Model file for the job. Use its own axes, mm. A direction names the side the tool comes from. Round coordinates to 2 decimals unless told otherwise and drop trailing zeros. Order: outer loops, then holes, each group sorted by start corner. A loop starts at its lowest first (then second) coordinate and runs counter-clockwise, first axis right, second up. Notation, with made-up numbers: (67, 57) -> (124, 57) arc R11 ccw to (124, 68) -> close; hole circle Ø10 at (-25.5, -33.5). An arc over 180 degrees is marked (long way). Put each result on its own line as item: value. Start each with the question number.
Q1. Cut at B-B, the plane z = 65.5. List the corners of the cut face in (x, y), and give its area (3 significant figures).
Q2. Probe L1, parallel to X at y = 1.9, z = 102; L2, parallel to X at y = 3.9, z = 28; L3, parallel to X at y = 3.2, z = 30. List the from-to ranges inside material, lowest first.
Q3. 3-axis set-ups, long thin cutter, end or side, ignore diameter. For faces 1 (the face through (-68, 2, 103.42)), 2 (the face through (-9.322, 2, 33)), 3 (the face through (-12.03, 2.46, 62.26)): which of +Z, -Z, +X, -X, +Y, -Y reach the whole face in a straight line?
Q4. Flat gauge pins, fed straight in: P1, Ø1, axis at x = -29.5, y = 4.5, coming from the +Z side; P2, Ø1.8, axis at y = 2, z = 109.5, coming from the +X side; P3, Ø1, axis at y = 2.5, z = 110, coming from the -X side. Where does each tip first touch, or does it go through?
Q5. Pull direction X, two halves, no side cores. Call faces 4 (the face through (-67.7, 2.46, 113.81)), 5 (the face through (-57.123, 2.465, 114.506)), 6 (the face through (-74.334, 2.465, 116.045)): released by +X, released by -X, zero draft, split by the parting line, or undercut.
Q6. Cut at A-A, the plane x = -20. List the corners of the cut face in (y, z), and give its area (3 significant figures).
Q7. Cut at C-C, the plane y = 1.9. State how many separate pieces and enclosed holes the cut face has, and give its area (3 significant figures).
from build123d import *

# Parameters (mm, degrees)
SKETCH2_R           = 3.0000000000000018
SKETCH2_R_2         = 1.4999999999993736
SKETCH2_R_3         = 1.5000000000000009
SKETCH2_R_4         = 1.4999999999993723
BOSS_EXTRUDE1_DEPTH = 5
FILLET1_R           = 1.5
FILLET3_R           = 10
FILLET5_R           = 10
CHAMFER1_SIZE       = 4.5
FILLET6_R           = 6
FILLET7_R           = 4
FILLET8_R           = 2
FILLET9_R           = 30
FILLET10_R          = 1


with BuildPart() as part:
    # Sketch2 → Boss-Extrude1 (new body)
    with BuildSketch(Plane(origin=(0, 0, 0), x_dir=(1, 0, 0), z_dir=(0, 1, 0))):
        with BuildLine():
            Line((-46.189355852298796, -96.42025186017804), (-39.496927389393186, -89.72782339727232))
            Line((-39.496927389393186, -89.72782339727232), (17.913506363615255, -32.31738964426288))
            Line((17.913506363615255, -32.31738964426288), (24.678224989376695, -32.31738964426288))
            Line((24.678224989376695, -32.31738964426288), (24.678224989376428, -17.06738964426295))
            Line((24.678224989376428, -17.06738964426295), (-7.595965049770856, -17.06738964426337))
            Line((-7.595965049770856, -17.06738964426337), (-7.595965049770857, -24.067389644263372))
            Line((-7.595965049770857, -24.067389644263372), (-9.321775010623746, -27.06012368042446))
            Line((-9.321775010623746, -27.06012368042446), (-9.32177501062375, -37.06738964426337))
            Line((-9.32177501062375, -37.06738964426337), (-9.321775010623757, -42.58210827002507))
            Line((-9.321775010623753, -42.58210827002507), (-54.6598701272448, -87.9202033866469))
            Line((-54.6598701272448, -87.9202033866469), (-60.17458875300816, -87.92020338664692))
            ThreePointArc((-60.17458875300816, -87.92020338664692), (-63.00301587775435, -89.09177626190073), (-64.17458875300817, -91.92020338664692))
            Line((-64.17458875300817, -91.92020338664692), (-64.17458875300817, -97.92020338664689))
            Line((-64.17458875300817, -97.92020338664689), (-70.17458875301077, -97.92020338664689))
            ThreePointArc((-70.17458875301077, -97.92020338664689), (-72.6339398041774, -98.76558892412923), (-74.05374095021992, -100.9444071830841))
            Line((-74.05374095021992, -100.9444071830841), (-77.14515150148509, -113.23391188563446))
            Line((-77.14515150148509, -113.23391188563446), (-71.4882972519927, -118.89076613512684))
            Line((-71.4882972519927, -118.89076613512684), (-59.047429208957894, -115.75810794021132))
            ThreePointArc((-59.047429208957894, -115.75810794021132), (-56.9723521770992, -114.3172183869977), (-56.174588753010745, -111.92020338664949))
            Line((-56.174588753010745, -111.92020338664949), (-56.174588753010745, -105.92020338664949))
            Line((-56.174588753010745, -105.92020338664949), (-50.174588753008145, -105.92020338664949))
            ThreePointArc((-50.174588753008145, -105.92020338664949), (-47.34616162826196, -104.74863051139567), (-46.174588753008145, -101.92020338664949))
            Line((-46.174588753008145, -101.92020338664949), (-46.17464642427909, -101.89872393503671))
            Line((-46.17464642427909, -101.89872393503671), (-46.189355852298796, -96.42025186017804))
        make_face()
        Polygon((-70.26446914062754, -114.4577399969996), (-72.71257361922765, -112.00963551839949), (-71.33075600396296, -106.51639746436214), (-66.89210317428027, -106.51639746436214), (-64.77078283072062, -108.63771780792177), (-64.7707828307206, -113.0744087552009), align=None, mode=Mode.SUBTRACT)
        with BuildLine():
            ThreePointArc((-61.67458875301074, -108.42020338664949), (-60.17458875301075, -106.92020338664949), (-58.67458875301077, -108.42020338664949))
            Line((-58.67458875301077, -108.42020338664949), (-58.674588753010774, -111.92020338664949))
            ThreePointArc((-58.674588753010774, -111.92020338664949), (-60.17458875301075, -113.42020338664946), (-61.67458875301073, -111.92020338664949))
            Line((-61.67458875301073, -111.92020338664949), (-61.67458875301074, -108.42020338664949))
        make_face(mode=Mode.SUBTRACT)
        with BuildLine():
            ThreePointArc((-66.67458875301074, -100.42020338664692), (-65.17458875301071, -101.92020338664692), (-66.67458875301074, -103.42020338664692))
            Line((-66.67458875301074, -103.42020338664692), (-70.17458875301077, -103.42020338664692))
            ThreePointArc((-70.17458875301077, -103.42020338664692), (-71.67458875301075, -101.92020338664692), (-70.17458875301077, -100.42020338664692))
            Line((-70.17458875301077, -100.4202033866469), (-66.67458875301074, -100.4202033866469))
        make_face(mode=Mode.SUBTRACT)
        with Locations(Location((-60.174588753008145, -101.92020338664949, 0), (0, 0, 270))):
            Circle(SKETCH2_R, mode=Mode.SUBTRACT)
        with BuildLine():
            ThreePointArc((-53.67458875300815, -103.42020338664949), (-55.17458875300815, -101.92020338664949), (-53.67458875300815, -100.42020338664949))
            Line((-53.67458875300815, -100.42020338664949), (-50.174588753008145, -100.42020338664949))
            ThreePointArc((-50.174588753008145, -100.42020338664949), (-48.67458875300816, -101.92020338664949), (-50.174588753008145, -103.42020338664949))
            Line((-50.174588753008145, -103.42020338664949), (-53.67458875300815, -103.42020338664949))
        make_face(mode=Mode.SUBTRACT)
        with BuildLine():
            ThreePointArc((-58.67458875300815, -95.42020338664692), (-60.17458875300815, -96.9202033866469), (-61.67458875300815, -95.42020338664692))
            Line((-61.674588753008145, -95.42020338664692), (-61.67458875300816, -91.92020338664692))
            ThreePointArc((-61.67458875300816, -91.92020338664692), (-60.174588753008145, -90.42020338664689), (-58.67458875300813, -91.92020338664692))
            Line((-58.67458875300813, -91.92020338664692), (-58.674588753008145, -95.42020338664692))
        make_face(mode=Mode.SUBTRACT)
        with Locations(Location((-1.1783767284213562, -42.92399136206118, 0), (0, 0, 270))):
            Circle(SKETCH2_R_2, mode=Mode.SUBTRACT)
        with Locations(Location((-3.3217750106237407, -28.067389644263372, 0), (0, 0, 270))):
            Circle(SKETCH2_R_3, mode=Mode.SUBTRACT)
        with Locations(Location((9.428224989376764, -32.31738964426288, 0), (0, 0, 270))):
            Circle(SKETCH2_R_4, mode=Mode.SUBTRACT)
        Polygon((1.0820753752795897, -25.575281589539195), (-1.459873180493811, -22.79599601598655), (-1.4598731804937872, -21.06738964426295), (17.849797864630506, -21.06738964426295), (11.740910030340089, -27.17627747855337), (10.272484798754686, -26.22755837455273), align=None, mode=Mode.SUBTRACT)
    extrude(amount=BOSS_EXTRUDE1_DEPTH)

    # Fillet1
    # the kernel refuses this fillet: 1.5 mm, written as the material it adds along each edge
    with BuildSketch(Plane(origin=(1.0820753752795897, 0, 25.575281589539195), x_dir=(0.9974908468725838, 0, 0.07079555357093803), z_dir=(0, 1, 0))) as fillet1_piece_1:
        with BuildLine():
            CenterArc((FILLET1_R * 0.398900109333, FILLET1_R), FILLET1_R, 226.50587582859146, 43.4941241714086)
            Line((-FILLET1_R * 0.289380073746, FILLET1_R * 0.274555040282), (0, 0))
            Line((0, 0), (FILLET1_R * 0.398900109333, 0))
        make_face()
    extrude(amount=5)
    with BuildSketch(Plane(origin=(-1.459873180493811, 0, 22.79599601598655), x_dir=(1.372e-14, 0, -1), z_dir=(0, 1, 0))) as fillet1_piece_2:
        with BuildLine():
            CenterArc((FILLET1_R * 0.388338270451, -FILLET1_R), FILLET1_R, 89.99999999999997, 42.44619337739144)
            Line((-FILLET1_R * 0.286559260205, -FILLET1_R * 0.262088539786), (0, 0))
            Line((0, 0), (FILLET1_R * 0.388338270451, 0))
        make_face()
    extrude(amount=5)
    with BuildSketch(Plane(origin=(-1.459873180493787, 0, 21.06738964426295), x_dir=(1, 0, 0), z_dir=(0, 1, 0))) as fillet1_piece_3:
        with BuildLine():
            CenterArc((FILLET1_R, -FILLET1_R), FILLET1_R, 90, 89.99999999999918)
            Line((-2.087e-14, -FILLET1_R), (0, 0))
            Line((0, 0), (FILLET1_R, 0))
        make_face()
    extrude(amount=5)
    with BuildSketch(Plane(origin=(11.740910030340089, 0, 27.17627747855337), x_dir=(-0.839945220222329, 0, -0.5426711960530642), z_dir=(0, 1, 0))) as fillet1_piece_4:
        with BuildLine():
            CenterArc((FILLET1_R * 0.807844840446, -FILLET1_R), FILLET1_R, 89.99999999999994, 77.86566453571226)
            Line((-FILLET1_R * 0.169812603282, -FILLET1_R * 0.789795521639), (0, 0))
            Line((0, 0), (FILLET1_R * 0.807844840446, -3e-17))
        make_face()
    extrude(amount=5)
    with BuildSketch(Plane(origin=(17.849797864630506, 0, 21.06738964426295), x_dir=(-0.7071067811865475, 0, 0.7071067811865475), z_dir=(0, 1, 0))) as fillet1_piece_5:
        with BuildLine():
            CenterArc((FILLET1_R * 2.41421356237, -FILLET1_R), FILLET1_R, 89.99999999999994, 135.00000000000006)
            Line((FILLET1_R * 1.70710678119, -FILLET1_R * 1.70710678119), (0, 0))
            Line((0, 0), (FILLET1_R * 2.41421356237, 1e-17))
        make_face()
    extrude(amount=5)
    # the kernel refuses this fillet: 1.5 mm, written as the material it takes off along each edge
    with BuildSketch(Plane(origin=(10.27248479875469, -0.9630450228974294, 26.22755837455273), x_dir=(0.8399452202223279, 0, 0.5426711960530661), z_dir=(0, 1, 0))) as fillet1_2_piece_1:
        with BuildLine():
            CenterArc((FILLET1_R * 0.256812006106, -FILLET1_R), FILLET1_R, 90.00000000000006, 28.805982084511456)
            Line((-FILLET1_R * 0.225033157983, -FILLET1_R * 0.123743623222), (0, 0))
            Line((0, 0), (FILLET1_R * 0.256812006106, 2e-17))
        make_face()
    extrude(amount=6.92609004579486, mode=Mode.SUBTRACT)

    # Fillet3
    fillet3_edges = [part.edges().sort_by_distance(p)[0] for p in [
        (17.913506363615255, 2.5, 32.31738964426288),
    ]]
    fillet(fillet3_edges, radius=FILLET3_R)

    # Fillet5
    fillet5_edges = [part.edges().sort_by_distance(p)[0] for p in [
        (-9.321775010623755, 2.5, 42.58210827002507),
    ]]
    fillet(fillet5_edges, radius=FILLET5_R)

    # Chamfer1
    chamfer1_edges = [part.edges().sort_by_distance(p)[0] for p in [
        (-64.17458875300817, 2.5, 97.92020338664689),
        (-56.174588753010745, 2.5, 105.92020338664949),
    ]]
    chamfer(chamfer1_edges, length=CHAMFER1_SIZE)

    # Fillet6
    fillet6_edges = [part.edges().sort_by_distance(p)[0] for p in [
        (-64.17458875300817, 2.5, 93.42020338664689),
        (-68.67458875300817, 2.5, 97.92020338664689),
        (-56.174588753010745, 2.5, 110.42020338664949),
        (-51.674588753010745, 2.5, 105.92020338664949),
    ]]
    fillet(fillet6_edges, radius=FILLET6_R)

    # Fillet7
    fillet7_edges = [part.edges().sort_by_distance(p)[0] for p in [
        (-71.4882972519927, 2.5, 118.89076613512684),
        (-77.14515150148509, 2.5, 113.23391188563446),
    ]]
    fillet(fillet7_edges, radius=FILLET7_R)

    # Fillet8
    fillet8_edges = [part.edges().sort_by_distance(p)[0] for p in [
        (-72.71257361922765, 2.5, 112.00963551839949),
        (-70.26446914062754, 2.5, 114.4577399969996),
        (-64.7707828307206, 2.5, 113.0744087552009),
        (-64.77078283072062, 2.5, 108.63771780792177),
        (-66.89210317428027, 2.5, 106.51639746436214),
        (-71.33075600396296, 2.5, 106.51639746436214),
    ]]
    fillet(fillet8_edges, radius=FILLET8_R)

    # Fillet9
    fillet9_edges = [part.edges().sort_by_distance(p)[0] for p in [
        (-54.6598701272448, 2.5, 87.9202033866469),
        (-46.189355852298796, 2.5, 96.42025186017804),
    ]]
    fillet(fillet9_edges, radius=FILLET9_R)

    # Fillet10
    fillet10_edges = [part.edges().sort_by_distance(p)[0] for p in [
        (-7.595965049770856, 2.5, 17.06738964426337),
        (24.678224989376428, 2.5, 17.06738964426295),
        (24.678224989376695, 2.5, 32.31738964426288),
    ]]
    fillet(fillet10_edges, radius=FILLET10_R)


solid = part.part
Ans:
1. outline: (-32.24, 0) -> (-15.27, 0) -> (-15.27, 5) -> (-32.24, 5) -> close
1. area: 84.9 mm^2
2. L1: x = -74.32 to -71.67, -65.18 to -63.17, -57.18 to -55.17, -48.68 to -46.07
2. L2: x = -9.32 to -4.82, -1.82 to 24.68
2. L3: x = -9.32 to 24.68
3. face 1: +Y, -Y
3. face 2: -Z, -X, +Y, -Y
3. face 3: +Z, +X, +Y, -Y
4. P1: stops at z = 80.23
4. P2: stops at x = -54.35
4. P3: stops at x = -76.46
5. face 4: undercut
5. face 5: released by +X
5. face 6: released by -X
6. outline: (0, 53.26) -> (5, 53.26) -> (5, 70.23) -> (0, 70.23) -> close
6. area: 84.9 mm^2
7. separate pieces: 1
7. enclosed holes: 10
7. area: 1,960 mm^2
